Geometry: final body of the model. Coordinates: model frame, mm. A direction names the side the tool comes from. Coordinates: 2 decimals unless noted, no trailing zeros. Loops run counter-clockwise (first coordinate to the right, second up) from the corner with the lowest first, then second, coordinate; pieces in that order, holes last. Notation, with made-up numbers: (64, 10) - (82, 10) arc R27 cw to (82, 31) - close; hole circle Ø3 at (24.5, 17.25). An arc over 180 degrees is marked (long way). Write each question's results on one line, items separated by ' | '. Start each with the question number.
from build123d import *

# Parameters (mm, degrees)
SKETCH1_W           = 35
SKETCH1_H           = 20
BOSS_EXTRUDE1_DEPTH = 25
SKETCH2_R           = 7.875
CUT_EXTRUDE1_DEPTH  = 21
SKETCH3_R           = 1.75
CUT_EXTRUDE2_DEPTH  = 10
FILLET1_R           = 12


with BuildPart() as part:
    # Sketch1 → Boss-Extrude1 (new body)
    with BuildSketch(Plane(origin=(0, 0, 0), x_dir=(1, 0, 0), z_dir=(0, 1, 0))):
        with Locations((1.164675851, -0.855170824)):
            Rectangle(SKETCH1_W, SKETCH1_H)
    extrude(amount=BOSS_EXTRUDE1_DEPTH)

    # Sketch2 → Cut-Extrude1 (cut, through all)
    with BuildSketch(Plane.XY.offset(10.855170824)):
        with Locations((1.164675851, 12)):
            Circle(SKETCH2_R)
    extrude(amount=-CUT_EXTRUDE1_DEPTH, mode=Mode.SUBTRACT)

    # Sketch3 → Cut-Extrude2 (cut)
    with BuildSketch(Plane.XZ):
        with Locations((-8.335324149, 0.855170824)):
            Circle(SKETCH3_R)
        with Locations((10.664675851, 0.855170824)):
            Circle(SKETCH3_R)
    extrude(amount=-CUT_EXTRUDE2_DEPTH, mode=Mode.SUBTRACT)

    # Fillet1
    fillet1_edges = [part.edges().sort_by_distance(p)[0] for p in [
        (18.664675851, 25, 0.855170824),
        (-16.335324149, 25, 0.855170824),
    ]]
    fillet(fillet1_edges, radius=FILLET1_R)


solid = part.part
1) Section query D-D on x = -6. Output: boundary loops of the cut face in (y, z).
2) Pull-direction query (X, two-part tool) for faces 1 (the flat face through (1, 25, 1)), 2 (the flat face through (-8, 10, 1)), 3 (the cylindrical face through (15.056, 21.578, 0.715)); classes: released by +X, released by -X, zero draft, split by the parting line, or undercut.
3) Section query B-B on z = 8. Output: boundary loops of the cut face in (x, y) (3 decimals).
4) Section query A-A on y = 12. Output: boundary loops of the cut face in (x, z), and give its area (3 significant figures).
5) Material intervals for line 1 (X direction, y = 12.5, z = 2.5); line 2 (Z direction, x = 12, y = 3.5); line 3 (Y direction, x = -4, z = 0.25), sorted ascending. Write a range as [from, to].
6) Section query C-C on y = 7.75. Output: boundary loops of the cut face in (x, z).
7) Pin query (flat end, axial travel): pin 1 Ø5 at (x, y) = (-4.5, 13) entering from +Z; pin 2 Ø1 at (y, z) = (15.5, -2.5) entering from -X; pin 3 Ø3 at (x, z) = (10.66, 0.86) entering from -Y; pin 4 Ø5.5 at (x, z) = (-8.34, 0.86) entering from +Y. Return the tip coordinate at first contact, or that it passes through.
8) Access query for faces 4 (the flat face through (11, 10, 1)), 5 (the flat face through (-7, 12, -9.145)). Directions: +Z, -Z, +X, -X, +Y, -Y. A direction counts if a zero-diameter tool reaches every point of the face in a straight line with its end or side. Return the directions, or none.
Returned:
1) outline: (0, -9.14) - (8.73, -9.14) - (8.73, 10.86) - (0, 10.86) - close; (15.27, -9.14) - (24.88, -9.14) - (24.88, 10.86) - (15.27, 10.86) - close
2) face 1: zero draft | face 2: undercut | face 3: released by +X
3) outline: (-16.335, 0) - (18.665, 0) - (18.665, 13) arc R12 ccw to (6.665, 25) - (-4.335, 25) arc R12 ccw to (-16.335, 13) - close; hole circle Ø15.75 at (1.165, 12)
4) outline: (-16.34, -9.14) - (-6.71, -9.14) - (-6.71, 10.86) - (-16.34, 10.86) - close; (9.04, -9.14) - (18.66, -9.14) - (18.66, 10.86) - (9.04, 10.86) - close | area: 385 mm²
5) line 1: x = [-16.34, -6.69], [9.02, 18.66] | line 2: z = [-9.14, -0.28], [1.99, 10.86] | line 3: y = [0, 6.06], [17.94, 25]
6) outline: (-16.34, -9.14) - (-5.47, -9.14) - (-5.47, 10.86) - (-16.34, 10.86) - close; (7.79, -9.14) - (18.66, -9.14) - (18.66, 10.86) - (7.79, 10.86) - close; hole circle Ø3.5 at (-8.34, 0.86); hole circle Ø3.5 at (10.66, 0.86)
7) pin 1: stops at z = 10.86 | pin 2: stops at x = -16.17 | pin 3: stops at y = 10 | pin 4: stops at y = 24.93
8) face 4: -Y | face 5: -Z, +X, -X, +Y, -Y
